```python
from build123d import *

# Parameters (mm, degrees)
SKETCH1_W               = 24
SKETCH1_H               = 81.502166862
BOSS_EXTRUDE1_DEPTH     = 3
SKETCH2_R               = 1.65
CUT_EXTRUDE1_DEPTH      = 4
BOSS_EXTRUDE2_START     = -6
SKETCH3_W               = 12
SKETCH3_H               = 1
BOSS_EXTRUDE2_DEPTH     = 75.502167
CUT_EXTRUDE2_DEPTH      = 2
CUT_EXTRUDE2_DEPTH_BACK = 1.5
SKETCH6_W               = 24
SKETCH6_H               = 32.3
SKETCH6_R               = 8.5
BOSS_EXTRUDE3_DEPTH     = 8
SKETCH9_R               = 1.15
CUT_EXTRUDE3_DEPTH      = 5
CUT_EXTRUDE4_START      = -1
CUT_EXTRUDE4_DEPTH      = 1.8


with BuildPart() as part:
    # Sketch1 → Boss-Extrude1 (new body)
    with BuildSketch(Plane(origin=(0, 0, 0), x_dir=(1, 0, 0), z_dir=(0, 1, 0))):
        with Locations((12, 40.751083431)):
            Rectangle(SKETCH1_W, SKETCH1_H)
    extrude(amount=BOSS_EXTRUDE1_DEPTH)

    # Sketch2 → Cut-Extrude1 (cut, through all)
    with BuildSketch(Plane(origin=(0, 0, 0), x_dir=(1, 0, 0), z_dir=(0, 1, 0))):
        with Locations((3.5, 3)):
            Circle(SKETCH2_R)
        with Locations((12, 3)):
            Circle(SKETCH2_R)
        with Locations((20.5, 3)):
            Circle(SKETCH2_R)
        with Locations((3.5, 62)):
            Circle(SKETCH2_R)
        with Locations((20.5, 62)):
            Circle(SKETCH2_R)
    extrude(amount=CUT_EXTRUDE1_DEPTH, mode=Mode.SUBTRACT)

    # Sketch3 → Boss-Extrude2 (add)
    with BuildSketch(Plane.XY.offset(BOSS_EXTRUDE2_START)):
        with Locations((12, 3.5)):
            Rectangle(SKETCH3_W, SKETCH3_H)
    extrude(amount=-BOSS_EXTRUDE2_DEPTH)

    # Sketch4 → Cut-Revolve1 (revolve, cut)
    with BuildSketch(Plane(origin=(12, 0, 0), x_dir=(0, 0, -1), z_dir=(1, 0, 0))):
        Polygon((94.496458379, 36.241477716), (19.413701779, -88.89644995), (139.590265278, -88.89644995), (139.590265278, 36.241477716), align=None)
    revolve(axis=Axis((12, 0, 0), (0, 1, 0)), mode=Mode.SUBTRACT)

    # Sketch5 → Cut-Extrude2 (cut, two sides)
    with BuildSketch(Plane(origin=(0, 3, 0), x_dir=(1, 0, 0), z_dir=(0, 1, 0))) as cut_extrude2_sk:
        Polygon((15.290896534, 3), (13.645448267, 5.85), (10.354551733, 5.85), (8.709103466, 3), (10.354551733, 0.15), (13.645448267, 0.15), align=None)
        Polygon((23.790896534, 3), (22.145448267, 5.85), (18.854551733, 5.85), (17.209103466, 3), (18.854551733, 0.15), (22.145448267, 0.15), align=None)
        Polygon((6.790896534, 3), (5.145448267, 5.85), (1.854551733, 5.85), (0.209103466, 3), (1.854551733, 0.15), (5.145448267, 0.15), align=None)
        Polygon((6.35, 63.645448267), (3.5, 65.290896534), (0.65, 63.645448267), (0.65, 60.354551733), (3.5, 58.709103466), (6.35, 60.354551733), align=None)
        Polygon((23.35, 63.645448267), (20.5, 65.290896534), (17.65, 63.645448267), (17.65, 60.354551733), (20.5, 58.709103466), (23.35, 60.354551733), align=None)
    extrude(amount=CUT_EXTRUDE2_DEPTH, mode=Mode.SUBTRACT)
    extrude(cut_extrude2_sk.sketch, amount=-CUT_EXTRUDE2_DEPTH_BACK, mode=Mode.SUBTRACT)

    # Sketch6 → Boss-Extrude3 (add)
    with BuildSketch(Plane.XY):
        with Locations((12, 16.15)):
            Rectangle(SKETCH6_W, SKETCH6_H)
        with Locations((12, 17.5)):
            Circle(SKETCH6_R, mode=Mode.SUBTRACT)
    extrude(amount=BOSS_EXTRUDE3_DEPTH)

    # Sketch9 → Cut-Extrude3 (cut)
    with BuildSketch(Plane(origin=(0, 32.3, 0), x_dir=(1, 0, 0), z_dir=(0, 1, 0))):
        with Locations((3, -4)):
            Circle(SKETCH9_R)
        with Locations((12, -4)):
            Circle(SKETCH9_R)
        with Locations((21, -4)):
            Circle(SKETCH9_R)
    extrude(amount=-CUT_EXTRUDE3_DEPTH, mode=Mode.SUBTRACT)

    # Sketch10 → Cut-Extrude4 (cut)
    with BuildSketch(Plane(origin=(0, 32.3, 0), x_dir=(1, 0, 0), z_dir=(0, 1, 0)).offset(CUT_EXTRUDE4_START)):
        Polygon((3, -6.424871131), (5.1, -5.212435565), (5.1, -2.787564435), (3, -1.575128869), (0.9, -2.787564435), (0.9, -5.212435565), align=None)
        Polygon((12, -6.424871131), (14.1, -5.212435565), (14.1, -2.787564435), (12, -1.575128869), (9.9, -2.787564435), (9.9, -5.212435565), align=None)
        Polygon((21, -6.424871131), (23.1, -5.212435565), (23.1, -2.787564435), (21, -1.575128869), (18.9, -2.787564435), (18.9, -5.212435565), align=None)
    extrude(amount=-CUT_EXTRUDE4_DEPTH, mode=Mode.SUBTRACT)


solid = part.part
```
Design review of the part built by this model. Coordinates are the model's own, in mm. A direction names the side the tool comes from. Coordinates: 2 decimals unless noted, no trailing zeros. Loops run counter-clockwise (first coordinate to the right, second up) from the corner with the lowest first, then second, coordinate; pieces in that order, holes last. Notation, with made-up numbers: (-14, 65) - (16, 65) arc R9 cw to (16, 72) - close; hole circle Ø2 at (60.5, 68.25). An arc over 180 degrees is marked (long way). Use CSV: the item, a comma, the result in double quotes. Start each with the question number.
1) For pin 1 Ø2 at (y, z) = (2, -62) entering from -X; pin 2 Ø1.8 at (x, z) = (12, 4) entering from +Y; pin 3 Ø13 at (x, z) = (14.5, -26) entering from +Y; pin 4 Ø8 at (y, z) = (8.5, -24.5) entering from -X, all flat-tipped, find the tip position at first contact; note any pin that passes through.
2) Wall thickness on L1, parallel to Y at x = 12, z = 5.5; L2, parallel to X at y = 28, z = 4; L3, parallel to X at y = 0.55, z = -3: over which ranges is each line inside the solid? List them lowest first. Write a range as from..to.
3) The part is to be moulded in two halves that separate along X. For faces 1 (the flat face through (5.1, 30, 4)), 2 (the conical face through (12.17, 1.53, -73.67)), say which applies: +X half, -X half, draft (parallel to the pull), parting line (faces both ways), or undercut.
4) Consider section D-D on y = 22.5. Write out the cut boundary in (x, z).
5) Consider section A-A on y = 17.5. Write out the cut boundary in (x, z).
6) Consider section B-B on z = -62. Write out the cut boundary in (x, y).
7) Consider section C-C on z = -36. Write out the cut boundary in (x, y).
8) Tool access review of faces 3 (the flat face through (18.04, 2.26, -4.44)), 4 (the flat face through (22.065, 30.413, 2.19)), 5 (the cylindrical face through (3.285, 0.74, -4.636)): name each direction out of +Z, -Z, +X, -X, +Y, -Y from which nothing blocks a thin tool from reaching the whole face with its end or side.
Geometry says:
1,pin 1,"x = 0"
1,pin 2,"y = 27.3"
1,pin 3,"y = 4"
1,pin 4,"through"
2,L1,"0..9, 26..29.5, 31.3..32.3"
2,L2,"0..1.85, 4.15..10.85, 13.15..19.85, 22.15..24"
2,L3,"0..1.85, 5.15..10.35, 13.65..18.85, 22.15..24"
3,face 1,"undercut"
3,face 2,"parting line"
4,outline,"(0, 0) - (5.13, 0) - (5.13, 8) - (0, 8) - close; (18.87, 0) - (24, 0) - (24, 8) - (18.87, 8) - close"
5,outline,"(0, 0) - (3.5, 0) - (3.5, 8) - (0, 8) - close; (20.5, 0) - (24, 0) - (24, 8) - (20.5, 8) - close"
6,outline,"(0, 0) - (1.85, 0) - (1.85, 1.5) - (0.65, 1.5) - (0.65, 3) - (0, 3) - close; (5.15, 0) - (18.85, 0) - (18.85, 1.5) - (17.65, 1.5) - (17.65, 4) - (6.35, 4) - (6.35, 1.5) - (5.15, 1.5) - close; (22.15, 0) - (24, 0) - (24, 3) - (23.35, 3) - (23.35, 1.5) - (22.15, 1.5) - close"
7,outline,"(0, 0) - (24, 0) - (24, 3) - (18, 3) - (18, 4) - (6, 4) - (6, 3) - (0, 3) - close"
8,face 3,"+Y"
8,face 4,"none"
8,face 5,"+Y, -Y"
